```python
from build123d import *

# Parameters (mm, degrees)
EXTRUDE_1_DEPTH           = 25
SHELL_2_T                 = -3
SKETCH_3_R                = 2.5
EXTRUDE_4_DEPTH           = 20
CUT_EXTRUDE_4_DEPTH       = 212.557459677
CUT_EXTRUDE_4_DEPTH_BACK  = 212.557459677
SKETCH_4_R                = 1.5
CUT_EXTRUDE_10_DEPTH      = 5
CUT_EXTRUDE_10_DEPTH_BACK = 212.890440429


with BuildPart() as part:
    # 草图1 → 凸台-拉伸1 (new body)
    with BuildSketch(Plane.XY):
        with BuildLine():
            Line((-193.42519685, 70), (-168.42519685, 70))
            ThreePointArc((-168.42519685, 70), (-164.889662944, 68.535533906), (-163.42519685, 65))
            Line((-163.42519685, 65), (-163.42519685, 5))
            ThreePointArc((-163.42519685, 5), (-164.889662944, 1.464466094), (-168.42519685, 0))
            Line((-168.42519685, 0), (-193.42519685, 0))
            ThreePointArc((-193.42519685, 0), (-196.960730756, 1.464466094), (-198.42519685, 5))
            Line((-198.42519685, 5), (-198.42519685, 65))
            ThreePointArc((-198.42519685, 65), (-196.960730756, 68.535533906), (-193.42519685, 70))
        make_face()
    extrude(amount=EXTRUDE_1_DEPTH)

    # 抽壳2
    shell_2_openings = [part.faces().sort_by_distance(p)[0] for p in [
        (-180.92519685, 35, 25),
    ]]
    offset(amount=SHELL_2_T, openings=shell_2_openings, kind=Kind.INTERSECTION)

    # 草图3 → 凸台-拉伸4 (add)
    with BuildSketch(Plane.XY.offset(3)):
        with Locations((-192.656739456, 62.5)):
            Circle(SKETCH_3_R)
        with Locations((-192.656739456, 7.5)):
            Circle(SKETCH_3_R)
        with Locations((-169.193654245, 62.5)):
            Circle(SKETCH_3_R)
        with Locations((-169.193654245, 7.5)):
            Circle(SKETCH_3_R)
    extrude(amount=EXTRUDE_4_DEPTH)

    # 草图4 → 切除-拉伸4 (cut, two sides: drawn at the far end of the back side and taken through both)
    with BuildSketch(Plane.XY.offset(3).offset(-CUT_EXTRUDE_4_DEPTH_BACK)):
        with Locations((-192.656739456, 62.5)):
            Circle(SKETCH_4_R)
        with Locations((-169.193654245, 62.5)):
            Circle(SKETCH_4_R)
        with Locations((-169.193654245, 7.5)):
            Circle(SKETCH_4_R)
        with Locations((-192.656739456, 7.5)):
            Circle(SKETCH_4_R)
    extrude(amount=CUT_EXTRUDE_4_DEPTH + CUT_EXTRUDE_4_DEPTH_BACK, mode=Mode.SUBTRACT)

    # 草图6 → 切除-拉伸10 (cut, two sides: drawn at the far end of the back side and taken through both)
    with BuildSketch(Plane(origin=(0, 0, 0), x_dir=(1, 0, 0), z_dir=(0, 1, 0)).offset(-CUT_EXTRUDE_10_DEPTH_BACK)):
        Polygon((-180.92519685, -25), (-175.92519685, -25), (-175.92519685, -21), (-185.92519685, -21), (-185.92519685, -25), align=None)
    extrude(amount=CUT_EXTRUDE_10_DEPTH + CUT_EXTRUDE_10_DEPTH_BACK, mode=Mode.SUBTRACT)


solid = part.part
```
Geometry check sheet. Reference: the model listing, model coordinates, mm. A direction names the side the tool comes from. Round coordinates to 2 decimals unless told otherwise and drop trailing zeros. Loops run counter-clockwise (first coordinate to the right, second up) from the corner with the lowest first, then second, coordinate; pieces in that order, holes last. Notation, with made-up numbers: M 21.5,67.25 L 40.5,67.25 A19 ccw 40.5,103.25 Z; hole C 29,15 d10. An arc over 180 degrees is marked long. Return JSON: item names as keys, results as strings. Group by question number.
(1) Section check B-B, the plane x = -175. Enter the section's corners in (y, z).
(2) Set-up check for faces 1 (the face through (-198.425, 35, 12)), 2 (the face through (-194.824, 3.57, 13.846)), 3 (the face through (-175.925, 1, 23)): record each of +Z, -Z, +X, -X, +Y, -Y from which the full face is reachable in a straight line by a thin tool's end or side.
(3) Section check D-D, the plane y = 17.5. Enter the section's corners in (x, z), and give its area (3 significant figures).
(4) Section check C-C, the plane y = 7.5. Enter the section's corners in (x, z), and give its area (3 significant figures).
(5) Mould release check, pull along Y, two halves, no side actions. Record for faces 4 (the face through (-194.64, 60.98, 12.86)), 5 (the face through (-181, 70, 12)), 6 (the face through (-163.425, 35, 12)): pulls with the +Y half, pulls with the -Y half, needs draft (parallel to the pull), parting line crosses it, or undercut.
(6) Section check A-A, the plane z = 8. Give the number of separate pieces and of enclosed holes in the cut face, and give its area (3 significant figures).
(7) Scan lines: line 1 along Y through (x, z) = (-169, 12.25); line 2 along X through (y, z) = (60.5, 12); line 3 along X through (y, z) = (14.5, 15). Record each from-to range of solid material in increasing order. Write a range as [from, to].
(8) Go/stop test with flat-tipped pins: pin 1 (0.9 mm diameter, centred on x = -180.5, y = 1, fed in from +Z); pin 2 (3 mm diameter, centred on x = -174, y = 14.5, fed in from +Z); pin 3 (1.5 mm diameter, centred on x = -169.5, y = 63, fed in from +Z); pin 4 (2.5 mm diameter, centred on x = -192, y = 6.5, fed in from +Z). Record where each tip stops, or that it passes through.
Data:
{
 "1": {"outline": "M 0,0 L 70,0 L 70,25 L 67,25 L 67,3 L 3,3 L 3,25 L 0,25 Z"},
 "2": {"face 1": "+Z, -Z, -X, +Y, -Y", "face 2": "+Z", "face 3": "+Z, -Y"},
 "3": {"outline": "M -198.43,0 L -163.43,0 L -163.43,25 L -166.43,25 L -166.43,3 L -195.43,3 L -195.43,25 L -198.43,25 Z", "area": "237 mm²"},
 "4": {"outline": "M -198.43,0 L -194.16,0 L -194.16,23 L -195.16,23 L -195.16,3 L -195.43,3 L -195.43,25 L -198.43,25 Z; M -191.16,0 L -170.69,0 L -170.69,23 L -171.69,23 L -171.69,3 L -190.16,3 L -190.16,23 L -191.16,23 Z; M -167.69,0 L -163.43,0 L -163.43,25 L -166.43,25 L -166.43,3 L -166.69,3 L -166.69,23 L -167.69,23 Z", "area": "299 mm²"},
 "5": {"face 4": "undercut", "face 5": "pulls with the +Y half", "face 6": "needs draft"},
 "6": {"separate pieces": "5", "enclosed holes": "5", "area": "626 mm²"},
 "7": {"line 1": "[0, 3], [5.01, 6.01], [8.99, 9.99], [60.01, 61.01], [63.99, 64.99], [67, 70]", "line 2": "[-198.43, -195.43], [-194.16, -191.16], [-170.69, -167.69], [-166.43, -163.43]", "line 3": "[-198.43, -195.43], [-166.43, -163.43]"},
 "8": {"pin 1": "z = 21", "pin 2": "z = 3", "pin 3": "through", "pin 4": "z = 23"}
}
